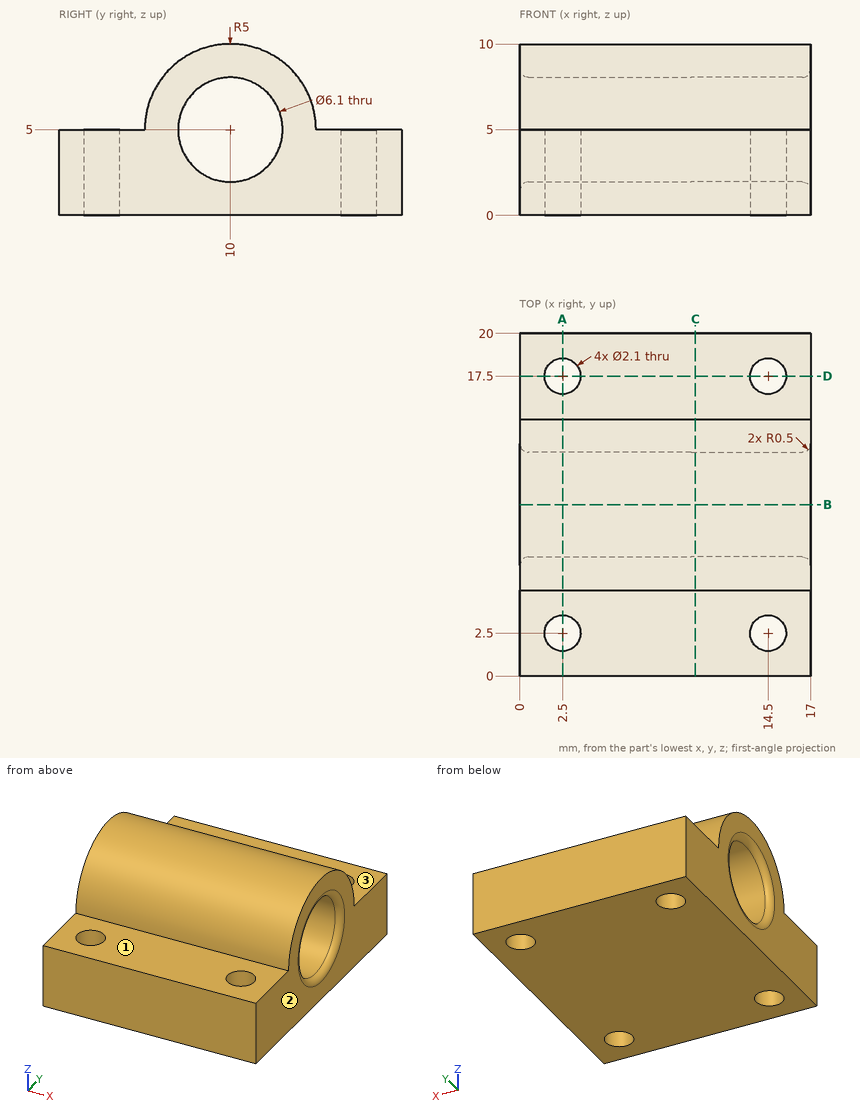
The figure shows three views and two pictorial views of one solid part (mm, origin at its lowest corner). Answer the questions. A direction names the side the tool comes from. Coordinates: 2 decimals unless noted, no trailing zeros. Order: outer loops, then holes, each group sorted by start corner. A loop starts at its lowest first (then second) coordinate and runs counter-clockwise, first axis right, second up.
Q1. A cutting plane is placed at B-B, the plane y = 10. Write down the section's boundary in (x, z).
Q2. Which of the six approach directions +Z, -Z, +X, -X, +Y, -Y give full straight-line access (tool end or side, diameter ignored) to the marked faces 1, 2 and 3?
Q3. A cutting plane is placed at D-D, the plane y = 17.5. Write down the section's boundary in (x, z).
Q4. Consider line 1 (X direction, y = 17.5, z = 3.4); line 2 (Z direction, x = 2.75, y = 10); line 3 (Y direction, x = 2.25, z = 4.75). Determine where each line is inside the solid, lowest interval first.
Q5. A cutting plane is placed at C-C, the plane x = 10.25. Write down the section's boundary in (y, z).
Q6. Given P1, Ø2.5, axis at x = 2.5, y = 2.5, coming from the -Z side; P2, Ø1, axis at x = 3.5, z = 7.5, coming from the +Y side; P3, Ø6, axis at x = 9.5, z = 8.5, coming from the -Y side; P4, Ø10, axis at x = 14.5, y = 18, coming from the +Z side, each flat-ended and moving along its own axis, determine where each tip first touches the part or whether it passes through.
Q7. A cutting plane is placed at A-A, the plane x = 2.5. Write down the section's boundary in (y, z), and give its area (3 significant figures).
Answers follow:
1. outline: (0, 0) - (17, 0) - (17, 1.45) arc R0.5 ccw to (16.5, 1.95) - (0.5, 1.95) arc R0.5 ccw to (0, 1.45) - close; (0, 8.55) arc R0.5 ccw to (0.5, 8.05) - (16.5, 8.05) arc R0.5 ccw to (17, 8.55) - (17, 10) - (0, 10) - close
2. face 1: +Z, +X, -X, -Y
2. face 2: +Z, -Z, +X, +Y, -Y
2. face 3: +Z, +X, -X, +Y
3. outline: (0, 0) - (1.45, 0) - (1.45, 5) - (0, 5) - close; (3.55, 0) - (13.45, 0) - (13.45, 5) - (3.55, 5) - close; (15.55, 0) - (17, 0) - (17, 5) - (15.55, 5) - close
4. line 1: x = 0 to 1.45, 3.55 to 13.45, 15.55 to 17
4. line 2: z = 0 to 1.95, 8.05 to 10
4. line 3: y = 0 to 1.48, 3.52 to 6.96, 13.04 to 16.48, 18.52 to 20
5. outline: (0, 0) - (20, 0) - (20, 5) - (15, 5) arc R5 ccw to (5, 5) - (0, 5) - close; hole circle Ø6.1 at (10, 5)
6. P1: stops at z = 0
6. P2: stops at y = 14.58
6. P3: stops at y = 5.03
6. P4: stops at z = 9
7. outline: (0, 0) - (1.45, 0) - (1.45, 5) - (0, 5) - close; (3.55, 0) - (16.45, 0) - (16.45, 5) - (15, 5) arc R5 ccw to (5, 5) - (3.55, 5) - close; (18.55, 0) - (20, 0) - (20, 5) - (18.55, 5) - close; hole circle Ø6.1 at (10, 5)
7. area: 89.0 mm2
